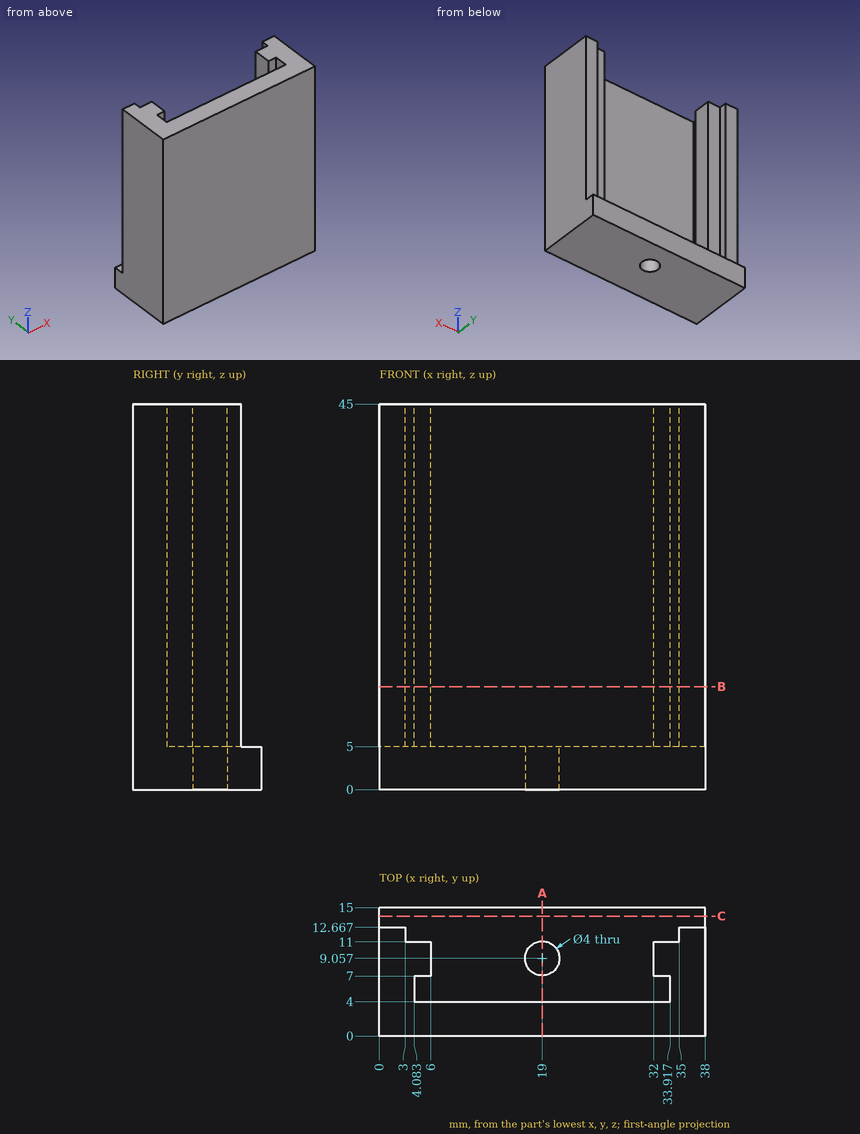
Check sheet for the drawn part. Datum: minimum x, y, z corner. Units: mm. Give positions to 0.01 mm unless a question says otherwise; leave off trailing zeros. Write each loop counter-clockwise with the first axis right and the second up, starting at its lowest first coordinate (ties: lowest second). Pieces come first, ordered by that corner, then holes. Notation, with made-up numbers: (43, 60) -> (74, 60) arc R19 ccw to (74, 74) -> close; hole circle Ø9 at (-39, -31.5). An arc over 180 degrees is marked (long way). Use one line per item in the form item = value. Start each with the question number.
1. Section check B-B (z = 12). Record the cut outline in (x, y).
2. Section check A-A (x = 19). Record the cut outline in (y, z).
3. Thickness scan on line 1 along Y through (x, z) = (19, 3); line 2 along X through (y, z) = (5.25, 40); line 3 along X through (y, z) = (9.5, 24). Record the ranges inside material, lowest first. Write a range as from..to.
4. Go/stop test with flat-tipped pins: P1, Ø3, axis at x = 9.5, z = 20.5, coming from the +Y side; P2, Ø0.9, axis at x = 4.5, z = 21, coming from the +Y side; P3, Ø5.5, axis at x = 12.5, y = 12, coming from the +Z side. Record where each tip stops, or that it passes through.
5. Section check C-C (y = 14). Record the cut outline in (x, z), and give its area (3 significant figures).
Conclusion:
q1.outline = (0, 0) -> (38, 0) -> (38, 12.67) -> (35, 12.67) -> (35, 11) -> (32, 11) -> (32, 7) -> (33.92, 7) -> (33.92, 4) -> (4.08, 4) -> (4.08, 7) -> (6, 7) -> (6, 11) -> (3, 11) -> (3, 12.67) -> (0, 12.67) -> close
q2.outline = (0, 0) -> (7.06, 0) -> (7.06, 5) -> (4, 5) -> (4, 45) -> (0, 45) -> close; (11.06, 0) -> (15, 0) -> (15, 5) -> (11.06, 5) -> close
q3.line_1 = 0..7.06, 11.06..15
q3.line_2 = 0..4.08, 33.92..38
q3.line_3 = 0..6, 32..38
q4.P1 = 4
q4.P2 = 11
q4.P3 = 5
q5.outline = (0, 0) -> (38, 0) -> (38, 5) -> (0, 5) -> close
q5.area = 190 mm²
